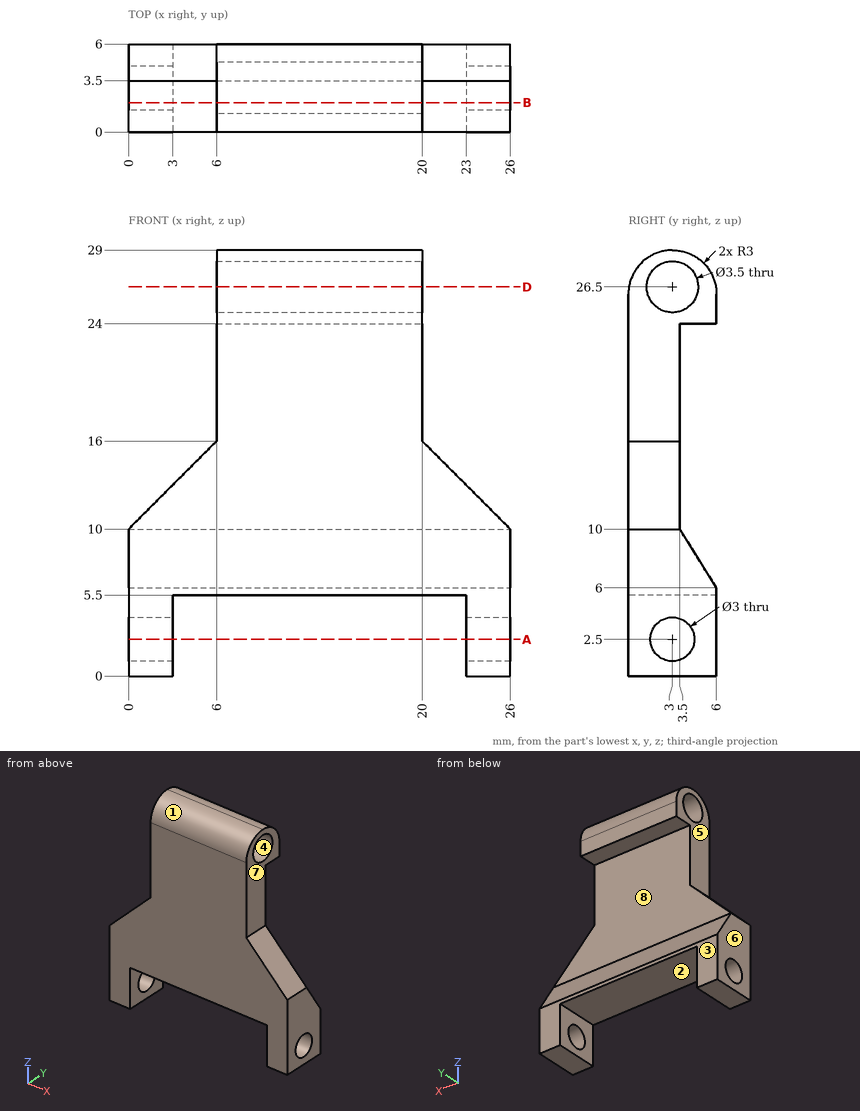
The figure shows three views and two pictorial views of one solid part (mm, origin at its lowest corner). Answer the questions. A direction names the side the tool comes from. Coordinates: 2 decimals unless noted, no trailing zeros. Order: outer loops, then holes, each group sorted by start corner. A loop starts at its lowest first (then second) coordinate and runs counter-clockwise, first axis right, second up.
Q1. Consider line 1 (Y direction, x = 23.75, z = 2.5); line 2 (X direction, y = 2.25, z = 4.5); line 3 (X direction, y = 3, z = 18.5). Determine where each line is inside the solid, lowest interval first.
Q2. Which of the six approach directions +Z, -Z, +X, -X, +Y, -Y give full straight-line access (tool end or side, diameter ignored) to the marked faces 5, 6, 7 and 8?
Q3. A cutting plane is placed at B-B, the plane y = 2. Write down the section's boundary in (x, z), and give its area (3 significant figures).
Q4. For a pull along Y with two mould halves and no side action, classify the marked faces 1, 2, 3 and 4 as pulls with the +Y half, pulls with the -Y half, needs draft (parallel to the pull), parting line crosses it, or undercut.
Q5. A cutting plane is placed at A-A, the plane z = 2.5. Write down the section's boundary in (x, y).
Q6. A cutting plane is placed at D-D, the plane z = 26.5. Write down the section's boundary in (x, y), and give its area (3 significant figures).
Q7. Given P1, Ø0.7, axis at x = 13.5, y = 4.5, coming from the -Z side; P2, Ø15.5, axis at x = 13.5, z = 15, coming from the +Y side, each flat-ended and moving along its own axis, determine where each tip first touches the part or whether it passes through.
Answers follow:
1. line 1: y = 0 to 1.5, 4.5 to 6
1. line 2: x = 0 to 3, 23 to 26
1. line 3: x = 6 to 20
2. face 5: +Z, -X, +Y, -Y
2. face 6: +Z, -Z, -X, +Y, -Y
2. face 7: +Z, +X, +Y, -Y
2. face 8: +X, -X, +Y
3. outline: (0, 0) - (3, 0) - (3, 1.38) - (0, 1.38) - close; (0, 3.62) - (3, 3.62) - (3, 5.5) - (23, 5.5) - (23, 3.62) - (26, 3.62) - (26, 10) - (20, 16) - (20, 25.06) - (6, 25.06) - (6, 16) - (0, 10) - close; (6, 27.94) - (20, 27.94) - (20, 28.83) - (6, 28.83) - close; (23, 0) - (26, 0) - (26, 1.38) - (23, 1.38) - close
3. area: 396 mm2
4. face 1: pulls with the -Y half
4. face 2: needs draft
4. face 3: pulls with the +Y half
4. face 4: undercut
5. outline: (0, 0) - (3, 0) - (3, 1.5) - (0, 1.5) - close; (0, 4.5) - (3, 4.5) - (3, 6) - (0, 6) - close; (23, 0) - (26, 0) - (26, 1.5) - (23, 1.5) - close; (23, 4.5) - (26, 4.5) - (26, 6) - (23, 6) - close
6. outline: (6, 0.04) - (20, 0.04) - (20, 1.25) - (6, 1.25) - close; (6, 4.75) - (20, 4.75) - (20, 5.96) - (6, 5.96) - close
6. area: 33.8 mm2
7. P1: stops at z = 5.5
7. P2: stops at y = 5.22
